Design review of the part built by this model. Coordinates are the model's own, in mm. Give positions to 0.01 mm unless a question says otherwise; leave off trailing zeros. Write each loop counter-clockwise with the first axis right and the second up, starting at its lowest first coordinate (ties: lowest second). Pieces come first, ordered by that corner, then holes.
```python
from build123d import *

# Parameters (mm, degrees)
EXTRUDE_1_DEPTH              = 3
SKETCH_2_R                   = 21.5
CUT_EXTRUDE_1_DEPTH          = 3
SKETCH_3_R                   = 1.525
CUT_EXTRUDE_2_DEPTH          = 3
FILLET_1_R                   = 3
SKETCH_4_R                   = 1.515
CUT_EXTRUDE_3_DEPTH          = 10
HOLE_WIZARD_M3_1_D           = 3
HOLE_WIZARD_M3_1_DEPTH       = 7.25
HOLE_WIZARD_M3_1_CSINK_D     = 6.6
HOLE_WIZARD_M3_1_CSINK_ANGLE = 90
HOLE_WIZARD_M3_1_TIP         = 0.901290929


with BuildPart() as part:
    # 草图1 → 凸台-拉伸1 (new body)
    with BuildSketch(Plane.XY):
        with BuildLine():
            Line((-20, -45), (20, -45))
            Line((20, -45), (27.083419191, -4.76848036))
            ThreePointArc((27.083419191, -4.76848036), (0, 27.5), (-27.083419191, -4.76848036))
            Line((-27.083419191, -4.76848036), (-20, -45))
        make_face()
    extrude(amount=EXTRUDE_1_DEPTH)

    # 草图2 → 切除-拉伸1 (cut)
    with BuildSketch(Plane.XY.offset(3)):
        Circle(SKETCH_2_R)
    extrude(amount=-CUT_EXTRUDE_1_DEPTH, mode=Mode.SUBTRACT)

    # 草图3 → 切除-拉伸2 (cut)
    with BuildSketch(Plane.XY.offset(3)):
        with Locations((17.324116139, 17.324116139)):
            Circle(SKETCH_3_R)
        with Locations((24.5, 0)):
            Circle(SKETCH_3_R)
        with Locations((17.324116139, -17.324116139)):
            Circle(SKETCH_3_R)
        with Locations((0, -24.5)):
            Circle(SKETCH_3_R)
        with Locations((-17.324116139, -17.324116139)):
            Circle(SKETCH_3_R)
        with Locations((-24.5, 0)):
            Circle(SKETCH_3_R)
        with Locations((-17.324116139, 17.324116139)):
            Circle(SKETCH_3_R)
        with Locations((0, 24.5)):
            Circle(SKETCH_3_R)
    extrude(amount=-CUT_EXTRUDE_2_DEPTH, mode=Mode.SUBTRACT)

    # 圆角1
    fillet_1_edges = [part.edges().sort_by_distance(p)[0] for p in [
        (20, -45, 1.5),
        (-20, -45, 1.5),
    ]]
    fillet(fillet_1_edges, radius=FILLET_1_R)

    # 草图4 → 切除-拉伸3 (cut)
    with BuildSketch(Plane.XY.offset(3)):
        with Locations((-15, -42)):
            Circle(SKETCH_4_R)
        with Locations((5, -42)):
            Circle(SKETCH_4_R)
    extrude(amount=-CUT_EXTRUDE_3_DEPTH, mode=Mode.SUBTRACT)

    # M3 十字槽沉头木螺钉的锥形沉头孔1
    with Locations(Plane.XY.offset(3)):
        with Locations((-15, -42), (5, -42)):
            CounterSinkHole(HOLE_WIZARD_M3_1_D / 2, HOLE_WIZARD_M3_1_CSINK_D / 2, depth=HOLE_WIZARD_M3_1_DEPTH, counter_sink_angle=HOLE_WIZARD_M3_1_CSINK_ANGLE)
            with Locations((0, 0, -(HOLE_WIZARD_M3_1_DEPTH + HOLE_WIZARD_M3_1_TIP / 2))):  # 118° drill point
                Cone(0, HOLE_WIZARD_M3_1_D / 2, HOLE_WIZARD_M3_1_TIP, mode=Mode.SUBTRACT)


solid = part.part
```
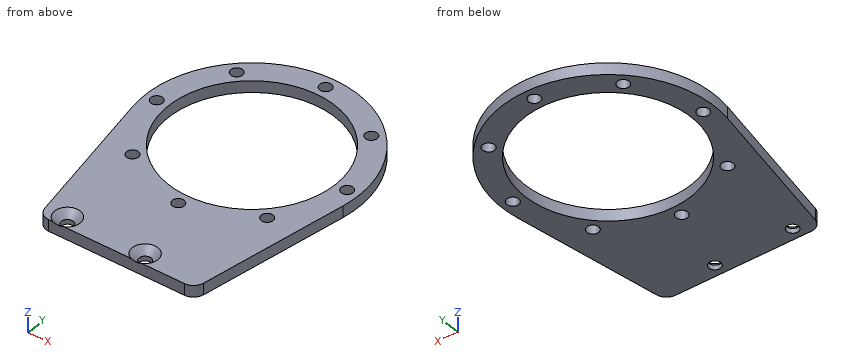
(1) To check wall thickness, follow L1, parallel to Y at x = 0.5, z = 2.3; L2, parallel to Y at x = -1, z = 1.9; L3, parallel to X at y = 17, z = 0.2. State the ranges of each line that lie inside material, in increasing order.
Resolved:
L1: y = -45 to -25.94, -23.06 to -21.49, 21.49 to 23.06, 25.94 to 27.5
L2: y = -45 to -25.65, -23.35 to -21.48, 21.48 to 23.35, 25.65 to 27.48
L3: x = -21.62 to -18.81, -15.83 to -13.16, 13.16 to 15.83, 18.81 to 21.62
(2) Consider section B-B, the plane x = 0. Give the boundary of the cut face in (y, z) (3 decimals).
Resolved:
outline: (-45, 0) - (-26.025, 0) - (-26.025, 3) - (-45, 3) - close; (-22.975, 0) - (-21.5, 0) - (-21.5, 3) - (-22.975, 3) - close; (21.5, 0) - (22.975, 0) - (22.975, 3) - (21.5, 3) - close; (26.025, 0) - (27.5, 0) - (27.5, 3) - (26.025, 3) - close
(3) Consider section C-C, the plane y = -11. Give the boundary of the cut face in (x, z).
Resolved:
outline: (-25.99, 0) - (-18.47, 0) - (-18.47, 3) - (-25.99, 3) - close; (18.47, 0) - (25.99, 0) - (25.99, 3) - (18.47, 3) - close
(4) Consider section A-A, the plane y = 0. Give the boundary of the cut face in (x, z) (3 decimals).
Resolved:
outline: (-27.5, 0) - (-26.025, 0) - (-26.025, 3) - (-27.5, 3) - close; (-22.975, 0) - (-21.5, 0) - (-21.5, 3) - (-22.975, 3) - close; (21.5, 0) - (22.975, 0) - (22.975, 3) - (21.5, 3) - close; (26.025, 0) - (27.5, 0) - (27.5, 3) - (26.025, 3) - close
(5) Consider section D-D, the plane z = 1.8. Give the number of separate pieces and of enclosed holes in the cut face, then the cut area to 3 significant figures.
Resolved:
separate pieces: 1
enclosed holes: 11
area: 1,800 mm2
(6) Clearance check with flat-ended pins moving along their axes: P1, Ø1, axis at x = -9, z = 1.5, coming from the +Y side; P2, Ø3.5, axis at x = 5, y = -42, coming from the +Z side. State where each tip first meets the part, or that it passes through.
Resolved:
P1: stops at y = 26.15
P2: stops at z = 1.45
